Work out the finished part from the listing and answer in its coordinate system (mm). Face numbers are marked on the shaded views. A direction names the side the tool comes from. Give positions to 0.01 mm unless a question says otherwise; leave off trailing zeros. Loops run counter-clockwise (first coordinate to the right, second up) from the corner with the lowest first, then second, coordinate; pieces in that order, holes last. Notation, with made-up numbers: M 85,60 L 102,60 A17 ccw 102,66 Z; hole C -0.5,86.25 d8. An arc over 180 degrees is marked long. Write item = value, one per line. Start each with the question number.
1. The mould has two halves that part along Z. Classify the marked faces 3 and 4: released by +Z, released by -Z, zero draft, split by the parting line, or undercut.
2. Section B-B on y = -150.5 is taken. Determine the outline of the cut face in (x, z) (3 decimals), plus the area to 3 significant figures.
3. For the marked faces 1 and 2, determine the directions among +Z, -Z, +X, -X, +Y, -Y from which every point of the face is accessible in a straight line to the end or side of a thin tool.
4. Flat-ended cylindrical pins translate along their axes: pin 1 Ø1.5 at (y, z) = (-97.5, 108.5) entering from +X; pin 2 Ø3.5 at (y, z) = (-82.76, -115.26) entering from +X; pin 3 Ø5 at (y, z) = (-141.79, -5.69) entering from +X; pin 4 Ø2 at (x, z) = (180.5, -11) entering from +Y. Find the tip coordinate at first contact, or state that the pin passes through.
5. Section A-A on z = -86.5 is taken. Determine the outline of the cut face in (x, y) (3 decimals), plus the area to 3 significant figures.
6. Consider L1, parallel to Z at x = 180, y = 3.5; L2, parallel to Z at x = 181.25, y = 0; L3, parallel to Z at x = 181.5, y = -85. Determine where each line is inside the solid, lowest interval first. Write a range as [from, to].
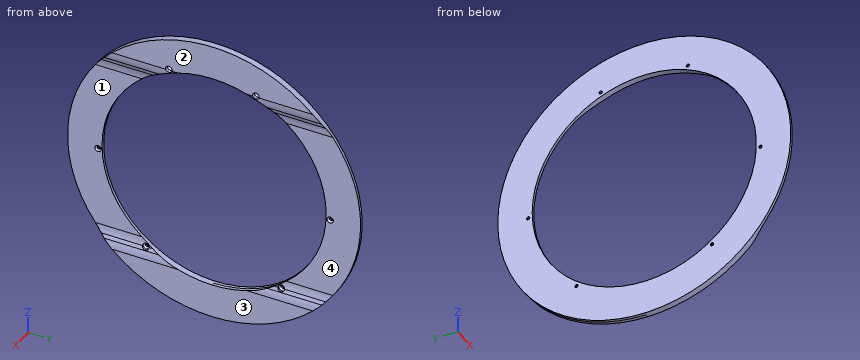
Autodesk Inventor part; units mm, degrees
ref_plane "XY Plane" through (0, 0, 0) normal (0, 0, 1) x (1, 0, 0)
ref_plane "Work Plane1" through (177.8, 0, 0) normal (1, 0, 0) x (0, 1, 0)
sketch "Sketch1" plane through (177.8, 0, 0) normal (1, 0, 0) x (0, 1, 0)
  circle A0 centre (0, 0) radius 178.9
  circle A1 centre (0, 0) radius 136.9
  dimension "d1" = 357.8
  dimension "d2" = 273.8
extrude "Extrusion1" add sketch "Sketch1" along normal blind 3.685
sketch "Sketch2" plane through (181.485, 0, 0) normal (1, 0, 0) x (0, 0, -1)
  line L0 (250.46, 0) -> (-250.46, 0) construction
  line L1 (0, -250.46) -> (0, 250.46) construction
  circle A0 centre (0, 0) radius 141.9 construction
  line L2 (0, 0) -> (-131.5488, 53.2026) construction
  line L3 (0, 0) -> (5.6947, 141.7857) construction
  line L4 (0, 0) -> (115.2635, 82.7643) construction
  point P0 (-131.5488, -53.2026)
  point P1 (5.6947, -141.7857)
  point P2 (115.2635, -82.7643)
  dimension "d5" = 283.8
  dimension "d6" = 22.02
  dimension "d7" = 92.3
  dimension "d8" = 144.32
hole "Hole1" at (181.485, 53.2026, 131.5488) at (181.485, 141.7857, -5.6947) at (181.485, 82.7643, -115.2635) at (181.485, -53.2026, 131.5488) at (181.485, -141.7857, -5.6947) at (181.485, -82.7643, -115.2635) direction (-1, 0, 0) diameter 4 end through all countersink diameter 8 countersink angle 90
sketch "Sketch3" plane through (181.485, 0, 0) normal (1, 0, 0) x (0, 0, -1)
  circle A0 centre (5.6947, -141.7857) radius 4
  circle A1 centre (115.2635, 82.7643) radius 4
  circle A2 centre (-131.5488, 53.2026) radius 4
  circle A3 centre (5.6947, 141.7857) radius 4
  circle A4 centre (-131.5488, -53.2026) radius 4
  circle A5 centre (115.2635, -82.7643) radius 4
  circle A6 centre (0, 0) radius 136.9
  circle A7 centre (0, 0) radius 178.9
extrude "Extrusion2" add sketch "Sketch3" along normal blind 4
sketch "Sketch4" plane through (0, 0, 0) normal (0, 1, 0) x (-1, 0, 0)
  line L0 (-185.485, 178.9) -> (-185.485, -178.9) construction
  line L1 (-177.8, -178.9) -> (-177.8, 178.9) construction
  line L2 (44.297, 0) -> (-265.782, 0) construction
  line L3 (-181.485, 0) -> (-181.485, 104.7583) construction
  line L4 (-185.485, 0) -> (-185.485, 125) construction
  line L5 (-182.8356, 115.0648) -> (-184.1344, 119.9352) construction
  arc A0 (-181.485, 104.7583) -> (-182.8356, 115.0648) centre (-221.485, 104.7583) ccw
  line L6 (-185.485, 130.2417) -> (-185.485, 178.9) construction
  arc A1 (-185.485, 130.2417) -> (-184.1344, 119.9352) centre (-145.485, 130.2417) ccw
  line L7 (-182.8356, 115.0648) -> (-184.1344, 119.9352)
  line L8 (-182.8356, -115.0648) -> (-184.1344, -119.9352) construction
  arc A2 (-182.8356, -115.0648) -> (-181.485, -104.7583) centre (-221.485, -104.7583) ccw
  arc A3 (-184.1344, -119.9352) -> (-185.485, -130.2417) centre (-145.485, -130.2417) ccw
  line L9 (-182.8356, -115.0648) -> (-184.1344, -119.9352)
  line L10 (-181.485, 104.7583) -> (-181.485, -104.7583)
  line L11 (-185.485, -130.2417) -> (-185.485, 130.2417)
  line L12 (-185.485, 127.5488) -> (-185.485, 135.5488)
  point P0 (0, 0)
  point P1 (-181.485, 110)
  dimension "d18" = 4
  dimension "d19" = 125
  dimension "d20" = 110
  dimension "d21" = 40
  dimension "d22" = 40
extrude "Extrusion3" cut sketch "Sketch4" along normal through all both and the other way through all
equation "\"d1\" = gxfront_OD"
equation "\"d2\" = gxfront_ID"
equation "\"d3\" = gxfront_t_total"
equation "\"d5\" = gxfront_d_holpos"
equation "\"d6\" = gxfront_a_hol_1"
equation "\"d7\" = gxfront_a_hol_2"
equation "\"d8\" = gxfront_a_hol_3"
equation "\"d9\" = gxfront_d_hol"
equation "\"d11\" = gxfront_d_holcs"
equation "\"d16\" = gxfront_t_extra"
equation "\"d18\" = gxfront_t_extra"
equation "\"d19\" = gxfront_z_extra"
equation "\"d21\" = gxfront_rfillet_zfair"
equation "\"d22\" = gxfront_rfillet_zfair"
equation "\"d23\" = gxfront_t_extra"
equation "\"gxfront_ID\" = 273.8"
equation "\"gxfront_OD\" = 357.8"
equation "\"gxfront_xbot\" = 177.8"
equation "\"gxfront_tbase\" = 1"
equation "\"gxfront_w_wire\" = 1.074"
equation "\"gxfront_t_total\" = 3.685"
equation "\"gxfront_d_holpos\" = 283.8"
equation "\"gxfront_d_hol\" = 4"
equation "\"gxfront_a_hol_1\" = 22.02deg"
equation "\"gxfront_a_hol_2\" = 92.3deg"
equation "\"gxfront_a_hol_3\" = 144.32deg"
equation "\"d0\" = gxfront_xbot"
equation "\"gxfront_d_holcs\" = 8"
equation "\"gxfront_z_extra\" = 125"
equation "\"gxfront_z_flat\" = 110"
equation "\"gxfront_t_extra\" = 4"
equation "\"gxfront_rfillet_zfair\" = 40"
equation "\"gxfront_t_total_offset\" = 0.5"
properties part number "GxFrontplate_base_191210_v02"
Verdict:
q1.face_3 = zero draft
q1.face_4 = undercut
q2.outline = M 177.8,-96.721 L 181.485,-96.721 L 181.485,96.721 L 177.8,96.721 Z
q2.area = 713 mm2
q3.face_1 = +X, +Y, -Y
q3.face_2 = +Z, -Z, +X, +Y, -Y
q4.pin_1 = 181.74
q4.pin_2 = through
q4.pin_3 = 179.99
q4.pin_4 = 178.62
q5.outline = M 177.8,-156.598 L 181.485,-156.598 L 181.485,-106.11 L 177.8,-106.11 Z; M 177.8,106.11 L 181.485,106.11 L 181.485,156.598 L 177.8,156.598 Z
q5.area = 372 mm2
q6.L1 = [-178.87, -136.86], [136.86, 178.87]
q6.L2 = [-178.9, -136.9], [136.9, 178.9]
q6.L3 = [-157.42, -118.58], [-111.95, -107.32], [107.32, 157.42]
